```python
from build123d import *

# Parameters (mm, degrees)
SKETCH2_W          = 55
SKETCH2_H          = 5
CUT_EXTRUDE1_DEPTH = 10
SKETCH3_W          = 70
SKETCH3_H          = 5
CUT_EXTRUDE2_DEPTH = 23
CHAMFER1_SIZE      = 1


with BuildPart() as part:
    # Sketch1 → Revolve1 (revolve)
    with BuildSketch(Plane.XY):
        Polygon((20, -138.5), (25, -138.5), (25, 0), (20, 0), (20, 58), (15, 58), (15, -50), (20, -50), align=None)
    revolve(axis=Axis((0, 0, 0), (0, 1, 0)))

    # Sketch2 → Cut-Extrude1 (cut)
    with BuildSketch(Plane(origin=(0, 58, 0), x_dir=(1, 0, 0), z_dir=(0, 1, 0))):
        Rectangle(SKETCH2_W, SKETCH2_H)
    extrude(amount=-CUT_EXTRUDE1_DEPTH, mode=Mode.SUBTRACT)

    # Sketch3 → Cut-Extrude2 (cut)
    with BuildSketch(Plane(origin=(0, -138.5, 0), x_dir=(-1, 0, 0), z_dir=(0, -1, 0))):
        Rectangle(SKETCH3_W, SKETCH3_H)
    extrude(amount=-CUT_EXTRUDE2_DEPTH, mode=Mode.SUBTRACT)

    # Chamfer1
    chamfer1_edges = [part.edges().sort_by_distance(p)[0] for p in [
        (0, 58, 15),
        (0, 58, -15),
        (0, 58, 20),
        (0, 58, -20),
        (0, -138.5, 25),
        (0, -138.5, -25),
        (0, -138.5, 20),
        (0, -138.5, -20),
        (-15, -50, 0),
        (-25, 0, 0),
    ]]
    chamfer(chamfer1_edges, length=CHAMFER1_SIZE)


solid = part.part
```
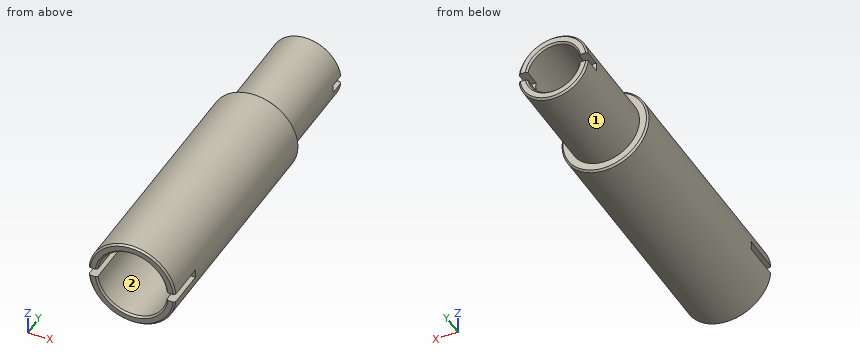
Geometry check sheet. Reference: the model listing, model coordinates, mm. Face numbers are marked on the shaded views. Give positions to 0.01 mm unless a question says otherwise; leave off trailing zeros. Order: outer loops, then holes, each group sorted by start corner. A loop starts at its lowest first (then second) coordinate and runs counter-clockwise, first axis right, second up. Notation, with made-up numbers: (81, 32.5) -> (90, 32.5) arc R23 cw to (90, 53.5) -> close; hole circle Ø10 at (10.5, -8.5). An arc over 180 degrees is marked (long way). Write each question's results on one line, items separated by ' | '. Start each with the question number.
(1) Sectioned sample at D-D (y = -99). Enter the section's corners in (x, z).
(2) Gauge pin test, flat ends, axial feed: P1, Ø4, axis at x = -9, z = 18.5, coming from the +Y side; P2, Ø4, axis at x = 16.5, y = 51, coming from the +Z side (3 decimals); P3, Ø1, axis at x = 19, y = -107, coming from the +Z side; P4, Ø1.5, axis at x = 23.5, y = -131, coming from the +Z side. Record the tip position at first contact, or that the pin passes through.
(3) Mould release check, pull along Z, two halves, no side actions. Record for the marked faces 1 and 2: pulls with the +Z half, pulls with the -Z half, needs draft (parallel to the pull), parting line crosses it, or undercut.
(4) Sectioned sample at A-A (x = 0). Enter the section's corners in (y, z), plus the area to 3 significant figures.
(5) Sectioned sample at B-B (z = 0). Enter the section's corners in (x, y).
(6) Scan lines: line 1 (X direction, y = -76, z = 0); line 2 (Z direction, x = -1, y = 18). Record each from-to range of solid material in increasing order.
(7) Sectioned sample at C-C (y = -120.5). Enter the section's corners in (x, z).
Answer below:
1) outline: circle Ø50 at (0, 0); hole circle Ø40 at (0, 0)
2) P1: y = 58 | P2: z = 13.775 | P3: z = 16.82 | P4: z = 10.37
3) face 1: parting line crosses it | face 2: undercut
4) outline: (-138.5, -24) -> (-137.5, -25) -> (-1, -25) -> (0, -24) -> (0, -20) -> (57, -20) -> (58, -19) -> (58, -16) -> (57, -15) -> (-49, -15) -> (-50, -16) -> (-50, -20) -> (-137.5, -20) -> (-138.5, -21) -> close; (-138.5, 21) -> (-137.5, 20) -> (-50, 20) -> (-50, 16) -> (-49, 15) -> (57, 15) -> (58, 16) -> (58, 19) -> (57, 20) -> (0, 20) -> (0, 24) -> (-1, 25) -> (-137.5, 25) -> (-138.5, 24) -> close | area: 2,460 mm2
5) outline: (-25, -115.5) -> (-20, -115.5) -> (-20, -50) -> (-16, -50) -> (-15, -49) -> (-15, 48) -> (-20, 48) -> (-20, 0) -> (-24, 0) -> (-25, -1) -> close; (15, -49) -> (16, -50) -> (20, -50) -> (20, -115.5) -> (25, -115.5) -> (25, -1) -> (24, 0) -> (20, 0) -> (20, 48) -> (15, 48) -> close
6) line 1: -25 to -20, 20 to 25 | line 2: -19.97 to -14.97, 14.97 to 19.97
7) outline: (-24.87, -2.5) arc R25 ccw to (24.87, -2.5) -> (19.84, -2.5) arc R20 cw to (-19.84, -2.5) -> close; (-24.87, 2.5) -> (-19.84, 2.5) arc R20 cw to (19.84, 2.5) -> (24.87, 2.5) arc R25 ccw to start
